from build123d import *

# Parameters (mm, degrees)
SKETCH_1_W          = 30
SKETCH_1_H          = 15
EXTRUDE_1_DEPTH     = 5
SKETCH_2_W          = 10
SKETCH_2_H          = 7.314170724
EXTRUDE_2_DEPTH     = 10
SKETCH_3_R          = 1.5
CUT_EXTRUDE_1_DEPTH = 6.5
SKETCH_4_W          = 4
SKETCH_4_H          = 7.314170724
CUT_EXTRUDE_2_DEPTH = 7
SKETCH_5_R          = 1.5
CUT_EXTRUDE_3_DEPTH = 15


with BuildPart() as part:
    # 草图1 → 凸台-拉伸1 (new body)
    with BuildSketch(Plane.XY):
        with Locations((15, 7.5)):
            Rectangle(SKETCH_1_W, SKETCH_1_H)
    extrude(amount=EXTRUDE_1_DEPTH)

    # 草图2 → 凸台-拉伸2 (add)
    with BuildSketch(Plane.XY.offset(5)):
        with Locations((15, 11.342914638)):
            Rectangle(SKETCH_2_W, SKETCH_2_H)
    extrude(amount=EXTRUDE_2_DEPTH)

    # 草图3 → 切除-拉伸1 (cut)
    with BuildSketch(Plane.XY.offset(5)):
        with Locations((5, 5)):
            Circle(SKETCH_3_R)
        with Locations((25, 5)):
            Circle(SKETCH_3_R)
    extrude(amount=-CUT_EXTRUDE_1_DEPTH, mode=Mode.SUBTRACT)

    # 草图4 → 切除-拉伸2 (cut)
    with BuildSketch(Plane.XY.offset(15)):
        with Locations((15, 11.342914638)):
            Rectangle(SKETCH_4_W, SKETCH_4_H)
    extrude(amount=-CUT_EXTRUDE_2_DEPTH, mode=Mode.SUBTRACT)

    # 草图5 → 切除-拉伸3 (cut)
    with BuildSketch(Plane.ZY.offset(-10)):
        with Locations(Location((12.5, 10, 0), (0, 0, 270))):
            Circle(SKETCH_5_R)
    extrude(amount=-CUT_EXTRUDE_3_DEPTH, mode=Mode.SUBTRACT)


solid = part.part
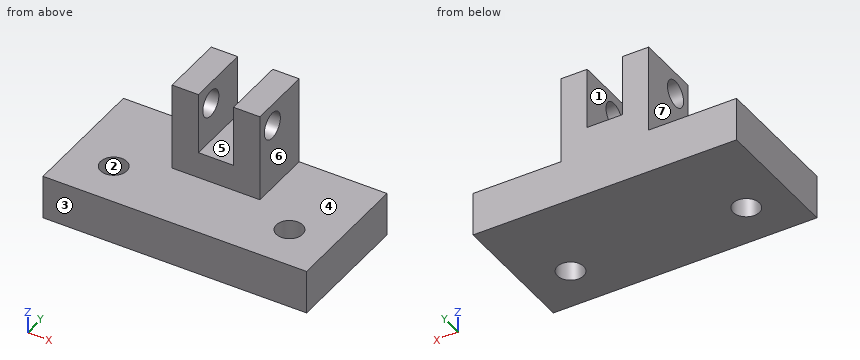
Check sheet for the modelled part. Datum: model origin and axes. Units: mm. Face numbers are marked on the shaded views. A direction names the side the tool comes from. Give positions to 0.01 mm unless a question says otherwise; leave off trailing zeros. Write each loop counter-clockwise with the first axis right and the second up, starting at its lowest first coordinate (ties: lowest second). Pieces come first, ordered by that corner, then holes. Notation, with made-up numbers: (-25, 25.25) -> (-8, 25.25) arc R9 ccw to (-8, 35.25) -> close; hole circle Ø9 at (-33.5, 32). An arc over 180 degrees is marked (long way). One line per item, written item: value. Start each with the question number.
Item 1: Section check C-C on x = 25. Record the cut outline in (y, z).
Item 2: Tool access check on the marked faces 4, 5, 6 and 7. Record the directions out of +Z, -Z, +X, -X, +Y, -Y that give a thin tool (end or side, any length) a straight path to the whole face; none if there is none.
Item 3: Section check D-D on z = 1.5. Record the cut outline in (x, y), then the cut area to 3 significant figures.
Item 4: Draft check along Y on the marked faces 1, 2 and 3. Enter one of: +Y half, -Y half, draft (parallel to the pull), parting line (faces both ways), or undercut.
Item 5: Section check B-B on z = 12.5. Record the cut outline in (x, y), then the cut area to 3 significant figures.
Item 6: Material ranges on probe 1 along Z at (x, y) = (18.7, 10); probe 2 along X at (y, z) = (9.5, 10); probe 3 along Z at (x, y) = (21, 2.5), recorded low to high. Write a range as from..to.
Item 7: Gauge pin test, flat ends, axial feed: pin 1 (5 mm diameter, centred on x = 23.5, y = 6, fed in from +Z); pin 2 (3.5 mm diameter, centred on y = 10.5, z = 8.5, fed in from +X); pin 3 (2 mm diameter, centred on y = 13, z = 10.5, fed in from -X). Record the tip position at first contact, or that the pin passes through.
Item 8: Section check A-A on y = 10. Record the cut outline in (x, z), then the cut area to 3 significant figures.
Results list:
1. outline: (0, 0) -> (3.5, 0) -> (3.5, 5) -> (0, 5) -> close; (6.5, 0) -> (15, 0) -> (15, 5) -> (6.5, 5) -> close
2. face 4: +Z, -Y
2. face 5: +Z, +Y, -Y
2. face 6: +Z, +X, +Y, -Y
2. face 7: +Z, -X, +Y, -Y
3. outline: (0, 0) -> (30, 0) -> (30, 15) -> (0, 15) -> close; hole circle Ø3 at (5, 5); hole circle Ø3 at (25, 5)
3. area: 436 mm²
4. face 1: draft
4. face 2: undercut
4. face 3: -Y half
5. outline: (10, 7.69) -> (13, 7.69) -> (13, 8.5) -> (10, 8.5) -> close; (10, 11.5) -> (13, 11.5) -> (13, 15) -> (10, 15) -> close; (17, 7.69) -> (20, 7.69) -> (20, 8.5) -> (17, 8.5) -> close; (17, 11.5) -> (20, 11.5) -> (20, 15) -> (17, 15) -> close
5. area: 25.9 mm²
6. probe 1: 0..11, 14..15
6. probe 2: 10..13, 17..20
6. probe 3: 0..5
7. pin 1: z = 5
7. pin 2: x = 20
7. pin 3: x = 10
8. outline: (0, 0) -> (30, 0) -> (30, 5) -> (20, 5) -> (20, 11) -> (17, 11) -> (17, 8) -> (13, 8) -> (13, 11) -> (10, 11) -> (10, 5) -> (0, 5) -> close; (10, 14) -> (13, 14) -> (13, 15) -> (10, 15) -> close; (17, 14) -> (20, 14) -> (20, 15) -> (17, 15) -> close
8. area: 204 mm²
